Autodesk Inventor part; units mm, degrees
ref_plane "YZ Plane" through (0, 0, 0) normal (1, 0, 0) x (0, 1, 0)
ref_plane "XZ Plane" through (0, 0, 0) normal (0, 1, 0) x (-1, 0, 0)
ref_plane "XY Plane" through (0, 0, 0) normal (0, 0, 1) x (1, 0, 0)
sketch "Sketch1" plane through (0, 0, 0) normal (0, 1, 0) x (-1, 0, 0)
  line L0 (147.3507, -0.6443) -> (74.3257, -0.6443)
  line L1 (74.3257, -0.6443) -> (74.3257, 50.1557)
  line L2 (74.3257, 50.1557) -> (147.3507, 50.1557)
  line L3 (147.3507, 50.1557) -> (147.3507, -0.6443)
  line L4 (147.3507, 50.1557) -> (142.5882, 50.1557)
  line L5 (142.5882, 50.1557) -> (142.5882, 46.9807)
  line L6 (142.5882, 46.9807) -> (147.3507, 46.9807)
  line L7 (147.3507, 46.9807) -> (147.3507, 50.1557)
  line L8 (129.8882, 50.1557) -> (117.1882, 50.1557)
  line L9 (117.1882, 50.1557) -> (117.1882, 46.9807)
  line L10 (117.1882, 46.9807) -> (129.8882, 46.9807)
  line L11 (129.8882, 46.9807) -> (129.8882, 50.1557)
  line L12 (104.4882, 50.1557) -> (91.7882, 50.1557)
  line L13 (91.7882, 50.1557) -> (91.7882, 46.9807)
  line L14 (91.7882, 46.9807) -> (104.4882, 46.9807)
  line L15 (104.4882, 46.9807) -> (104.4882, 50.1557)
  line L16 (147.3507, 2.5307) -> (147.3507, -0.6443)
  line L17 (129.8882, -0.6443) -> (117.1882, -0.6443)
  line L18 (104.4882, -0.6443) -> (91.7882, -0.6443)
  line L19 (147.3507, 8.8807) -> (147.3507, 15.2307)
  line L20 (147.3507, 15.2307) -> (144.1757, 15.2307)
  line L21 (144.1757, 15.2307) -> (144.1757, 8.8807)
  line L22 (144.1757, 8.8807) -> (147.3507, 8.8807)
  line L23 (147.3507, 21.5807) -> (147.3507, 27.9307)
  line L24 (147.3507, 27.9307) -> (144.1757, 27.9307)
  line L25 (144.1757, 27.9307) -> (144.1757, 21.5807)
  line L26 (144.1757, 21.5807) -> (147.3507, 21.5807)
  line L27 (147.3507, 34.2807) -> (147.3507, 40.6307)
  line L28 (147.3507, 40.6307) -> (144.1757, 40.6307)
  line L29 (144.1757, 40.6307) -> (144.1757, 34.2807)
  line L30 (144.1757, 34.2807) -> (147.3507, 34.2807)
  line L31 (74.3257, 46.9807) -> (74.3257, 50.1557)
  line L32 (74.3257, 2.5307) -> (74.3257, -0.6443)
  line L33 (79.0882, -0.6443) -> (79.0882, 2.5307)
  line L34 (79.0882, 2.5307) -> (91.7882, 2.5307)
  line L35 (91.7882, 2.5307) -> (91.7882, -0.6443)
  line L36 (91.7882, -0.6443) -> (79.0882, -0.6443)
  line L37 (104.4882, 2.5307) -> (104.4882, -0.6443)
  line L38 (104.4882, -0.6443) -> (117.1882, -0.6443)
  line L39 (117.1882, -0.6443) -> (117.1882, 2.5307)
  line L40 (117.1882, 2.5307) -> (104.4882, 2.5307)
  line L41 (129.8882, -0.6443) -> (129.8882, 2.5307)
  line L42 (129.8882, 2.5307) -> (142.5882, 2.5307)
  line L43 (142.5882, 2.5307) -> (142.5882, -0.6443)
  line L44 (142.5882, -0.6443) -> (129.8882, -0.6443)
  line L45 (74.3257, 50.1557) -> (74.3257, 18.4057)
  line L46 (74.3257, 46.9807) -> (74.3257, 50.1557)
  line L47 (79.0882, 50.1557) -> (66.3882, 50.1557)
  line L48 (66.3882, 50.1557) -> (66.3882, 46.9807)
  line L49 (66.3882, 46.9807) -> (79.0882, 46.9807)
  line L50 (79.0882, 46.9807) -> (79.0882, 50.1557)
  line L51 (66.3882, 50.1557) -> (63.2132, 50.1557)
  line L52 (63.2132, 50.1557) -> (63.2132, 46.9807)
  line L53 (63.2132, 46.9807) -> (66.3882, 46.9807)
  line L54 (66.3882, 46.9807) -> (66.3882, 50.1557)
  line L55 (63.2132, 50.1557) -> (31.4632, 50.1557)
  line L56 (31.4632, 50.1557) -> (31.4632, 38.1669)
  line L57 (31.4632, 38.1669) -> (63.2132, 38.1669)
  line L58 (63.2132, 38.1669) -> (63.2132, 50.1557)
  line L59 (63.2132, 46.9807) -> (63.2132, 50.1557)
  line L60 (63.2132, 50.1557) -> (31.4632, 50.1557)
  line L61 (31.4632, 50.1557) -> (31.4632, 46.9807)
  line L62 (31.4632, 46.9807) -> (63.2132, 46.9807)
  line L63 (31.4632, 50.1557) -> (34.6382, 50.1557)
  line L64 (34.6382, 50.1557) -> (34.6382, 46.9807)
  line L65 (34.6382, 46.9807) -> (31.4632, 46.9807)
  line L66 (31.4632, 46.9807) -> (31.4632, 50.1557)
  line L67 (74.3257, 46.9807) -> (55.2757, 46.9807)
  line L68 (55.2757, 46.9807) -> (55.2757, 9.5919)
  line L69 (55.2757, 9.5919) -> (74.3257, 9.5919)
  line L70 (74.3257, 9.5919) -> (74.3257, 46.9807)
  point P0 (0, 0)
  point P1 (79.0882, -0.6443)
  point P2 (91.7882, -0.6443)
  point P3 (104.4882, -0.6443)
  point P4 (117.1882, -0.6443)
  point P5 (129.8882, -0.6443)
  point P6 (142.5882, -0.6443)
  point P7 (55.2757, 38.1669)
  dimension "d103" = 73.025
  dimension "d105" = 4.7625
  dimension "d106" = 3.175
  dimension "d107" = 12.7
  dimension "d108" = 3.175
  dimension "d109" = 12.7
  dimension "d110" = 3.175
  dimension "d111" = 12.7
  dimension "d112" = 12.7
  dimension "d121" = 6.35
  dimension "d122" = 3.175
  dimension "d123" = 6.35
  dimension "d124" = 3.175
  dimension "d126" = 6.35
  dimension "d127" = 6.35
  dimension "d128" = 3.175
  dimension "d129" = 6.35
  dimension "d146" = 3.175
  dimension "d147" = 12.7
  dimension "d148" = 0
  dimension "d149" = 4.7625
  dimension "d150" = 3.175
  dimension "d151" = 12.7
  dimension "d152" = 12.7
  dimension "d153" = 0
  dimension "d154" = 3.175
  dimension "d155" = 12.7
  dimension "d156" = 12.7
  dimension "d161" = 0
  dimension "d168" = 12.7
  dimension "d169" = 3.175
  dimension "d170" = 12.7
  dimension "d171" = 3.175
  dimension "d172" = 3.175
  dimension "d182" = 31.75
  dimension "d183" = 11.9888
  dimension "d186" = 3.175
  dimension "d195" = 19.05
  dimension "d196" = 37.3888
extrude "Extrusion15" add sketch "Sketch1" along normal blind 25.4 contours L0 L43 L42 L41 L39 L40 L37 L35 L34 L33 L1 L49 L50 L2 L13 L14 L15 L9 L10 L11 L5 L6 L3 L28 L29 L30 L24 L25 L26 L20 L21 L22 | L69 L68 L57 L58 L53 L49 L1 | L68 L62 L58 L57 | L57 L56 L62 L68 | L53 L52 L51 L48 | L56 L55 L64 L62
equation "\"BendRadius\" = Thickness"
equation "\"BendReliefWidth\" = Thickness"
equation "\"BendReliefDepth\" = 0.5 * Thickness"
equation "\"CornerReliefSize\" = 4 * Thickness"
equation "\"MinimumRemnant\" = 2 * Thickness"
equation "\"TransitionRadius\" = BendRadius"
equation "\"JacobiRadiusSize\" = BendRadius"
equation "\"GapSize\" = Thickness"
properties part number "V9_BURROW_SIDE"
The model under review builds one solid part; all positions refer to its coordinate system, in mm. A direction names the side the tool comes from. Round coordinates to 2 decimals unless told otherwise and drop trailing zeros. Write each loop counter-clockwise with the first axis right and the second up, starting at its lowest first coordinate (ties: lowest second). Pieces come first, ordered by that corner, then holes. Notation, with made-up numbers: M 28,64 L 56,64 A6 ccw 56,73 Z; hole C -14.75,-25 d2. An arc over 180 degrees is marked long. Use CSV: the item, a comma, the result in double quotes. Start each with the question number.
(1) We need section B-B, the plane x = -60.5. State the section outline as (y, z) points, then the cut area to 3 significant figures.
(2) Clearance check with flat-ended pins moving along their axes: P1, Ø1.6, axis at y = 7.5, z = 48, coming from the -X side; P2, Ø3, axis at y = 7.5, z = 12, coming from the -X side; P3, Ø5.5, axis at x = -63.5, y = 9, coming from the -Z side. State where each tip first meets the part, or that it passes through.
(3) We need section A-A, the plane z = 33. State the section outline as (x, y) points.
(4) For line 1 along X through (y, z) = (4.5, 2); line 2 along Z through (x, y) = (-70.5, 11); line 3 along Z through (x, y) = (-37.5, 23.25), list the stretches that pass through material, from the lowest coordinate up.
(5) The part is to be moulded in two halves that separate along X. For faces 1 (the face through (-144.176, 13, 12)), 2 (the face through (-117.188, 13, 49)), 3 (the face through (-74.326, 13, 4)), say which applies: +X half, -X half, draft (parallel to the pull), parting line (faces both ways), or undercut.
(6) Tool access review of faces 4 (the face through (-117.188, 13, 1)), 5 (the face through (-129.888, 13, 49)), 6 (the face through (-142.588, 13, 49)), 7 (the face through (-146, 13, 27.931)), 8 (the face through (-43, 13, 38.167)): name each direction out of +Z, -Z, +X, -X, +Y, -Y from which nothing blocks a thin tool from reaching the whole face with its end or side.
Findings:
1,outline,"M 0,9.59 L 25.4,9.59 L 25.4,46.98 L 0,46.98 Z"
1,area,"950 mm^2"
2,P1,"x = -142.59"
2,P2,"x = -144.18"
2,P3,"z = 9.59"
3,outline,"M -147.35,0 L -55.28,0 L -55.28,25.4 L -147.35,25.4 Z"
4,line 1,"-147.35 to -142.59, -129.89 to -117.19, -104.49 to -91.79, -79.09 to -74.33"
4,line 2,"9.59 to 46.98"
4,line 3,"38.17 to 46.98"
5,face 1,"-X half"
5,face 2,"undercut"
5,face 3,"+X half"
6,face 4,"-Z, +Y, -Y"
6,face 5,"+Z, +Y, -Y"
6,face 6,"+Z, -X, +Y, -Y"
6,face 7,"-X, +Y, -Y"
6,face 8,"-Z, +X, +Y, -Y"
